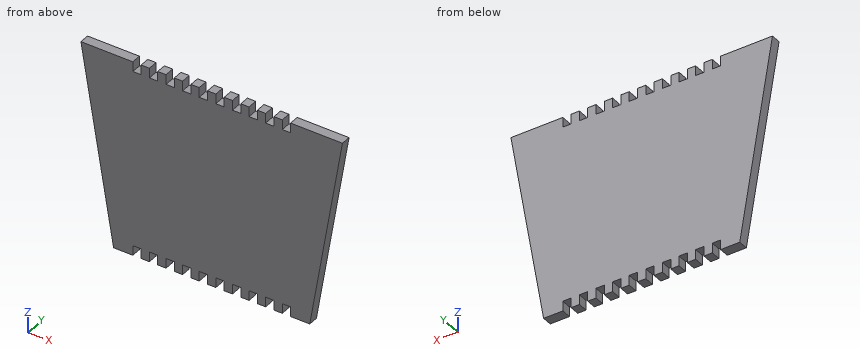
```python
from build123d import *

# Parameters (mm, degrees)
F1_DEPTH = 15


# Not quite as in the source:
# - a feature names something its author has since deleted; it is built from what else it names


with BuildPart() as f1:
    # F0 (on Front) → F1 (new body)
    with BuildSketch(Plane.XZ):
        Polygon((150, -150), (200, 150), (120.65, 150), (120.65, 135), (107.95, 135), (107.95, 150), (95.25, 150), (95.25, 135), (82.55, 135), (82.55, 150), (69.85, 150), (69.85, 135), (57.15, 135), (57.15, 150), (44.45, 150), (44.45, 135), (31.75, 135), (31.75, 150), (19.05, 150), (19.05, 135), (6.35, 135), (6.35, 150), (0, 150), (-6.35, 150), (-6.35, 135), (-19.05, 135), (-19.05, 150), (-31.75, 150), (-31.75, 135), (-44.45, 135), (-44.45, 150), (-57.15, 150), (-57.15, 135), (-69.85, 135), (-69.85, 150), (-82.55, 150), (-82.55, 135), (-95.25, 135), (-95.25, 150), (-107.95, 150), (-107.95, 135), (-120.65, 135), (-120.65, 150), (-200, 150), (-150, -150), (-120.65, -150), (-120.65, -135), (-107.95, -135), (-107.95, -150), (-95.25, -150), (-95.25, -135), (-82.55, -135), (-82.55, -150), (-69.85, -150), (-69.85, -135), (-57.15, -135), (-57.15, -150), (-44.45, -150), (-44.45, -135), (-31.75, -135), (-31.75, -150), (-19.05, -150), (-19.05, -135), (-6.35, -135), (-6.35, -150), (0, -150), (6.35, -150), (6.35, -135), (19.05, -135), (19.05, -150), (31.75, -150), (31.75, -135), (44.45, -135), (44.45, -150), (57.15, -150), (57.15, -135), (69.85, -135), (69.85, -150), (82.55, -150), (82.55, -135), (95.25, -135), (95.25, -150), (107.95, -150), (107.95, -135), (120.65, -135), (120.65, -150), align=None)
    extrude(amount=F1_DEPTH)


solid = f1.part
```
Could you check a few things on this model? Use its own coordinates, in mm. Round coordinates to 2 decimals unless told otherwise and drop trailing zeros. Loops run counter-clockwise (first coordinate to the right, second up) from the corner with the lowest first, then second, coordinate; pieces in that order, holes last. Notation, with made-up numbers: (14.25, 3.25) -> (65.25, 3.25) arc R16 cw to (65.25, 15.25) -> close; hole circle Ø2 at (-23.75, 18). An arc over 180 degrees is marked (long way). One line per question, with ' | ' between items.
(1) If I drill on probe 1 along Z at (x, y) = (-111, -1); probe 2 along X at (y, z) = (-7, -25); probe 3 along X at (y, z) = (-12.25, 15), over which ranges is the centre line in solid material (lowest first)?
Model answer:
probe 1: z = -135 to 135 | probe 2: x = -170.83 to 170.83 | probe 3: x = -177.5 to 177.5
(2) If we section it at B-B on x = 37: List the corners of the cut face in (y, z) for me.
Model answer:
outline: (-15, -135) -> (0, -135) -> (0, 135) -> (-15, 135) -> close
(3) For pin 1 Ø6.5 at (x, y) = (62.5, -4) entering from +Z; pin 2 Ø7.5 at (y, z) = (-4, 141) entering from -X (3 decimals); pin 3 Ø6.5 at (x, y) = (-39.5, -7) entering from -Z, each with a flat end and sliding along its axis, tell me the tip position at first contact or that it passes through.
Model answer:
pin 1: stops at z = 135 | pin 2: stops at x = -199.125 | pin 3: stops at z = -135
(4) If we section it at A-A on z = -75: List the corners of the cut face in (x, y) for me, and give its area (4 significant figures).
Model answer:
outline: (-162.5, -15) -> (162.5, -15) -> (162.5, 0) -> (-162.5, 0) -> close | area: 4,875 mm^2
